from build123d import *

# Parameters (mm, degrees)
SKETCH1_R                   = 13
BOSS_EXTRUDE1_DEPTH         = 3.5
SKETCH2_R                   = 20
BOSS_EXTRUDE2_DEPTH         = 1
SKETCH3_R                   = 26
BOSS_EXTRUDE3_DEPTH         = 1
SKETCH4_R                   = 23.03
BOSS_EXTRUDE4_DEPTH         = 7.5
SKETCH5_R                   = 26
BOSS_EXTRUDE5_DEPTH         = 1
SKETCH6_R                   = 20
BOSS_EXTRUDE6_DEPTH         = 1
SKETCH7_R                   = 11
CUT_EXTRUDE1_DEPTH          = 40.711459303
TAP_DRILL_FOR_M3X0_5_TAP1_D = 3.4
CHAMFER1_SIZE               = 0.5


with BuildPart() as part:
    # Sketch1 → Boss-Extrude1 (new body)
    with BuildSketch(Plane.XY):
        Circle(SKETCH1_R)
    extrude(amount=BOSS_EXTRUDE1_DEPTH)

    # Sketch2 → Boss-Extrude2 (add)
    with BuildSketch(Plane.XY.offset(3.5)):
        Circle(SKETCH2_R)
    extrude(amount=BOSS_EXTRUDE2_DEPTH)

    # Sketch3 → Boss-Extrude3 (add)
    with BuildSketch(Plane.XY.offset(4.5)):
        Circle(SKETCH3_R)
    extrude(amount=BOSS_EXTRUDE3_DEPTH)

    # Sketch4 → Boss-Extrude4 (add)
    with BuildSketch(Plane.XY.offset(5.5)):
        Circle(SKETCH4_R)
    extrude(amount=BOSS_EXTRUDE4_DEPTH)

    # Sketch5 → Boss-Extrude5 (add)
    with BuildSketch(Plane.XY.offset(13)):
        Circle(SKETCH5_R)
    extrude(amount=BOSS_EXTRUDE5_DEPTH)

    # Sketch6 → Boss-Extrude6 (add)
    with BuildSketch(Plane.XY.offset(14)):
        Circle(SKETCH6_R)
    extrude(amount=BOSS_EXTRUDE6_DEPTH)

    # Sketch7 → Cut-Extrude1 (cut, through all)
    with BuildSketch(Plane.XY.offset(15)):
        Circle(SKETCH7_R)
    extrude(amount=-CUT_EXTRUDE1_DEPTH, mode=Mode.SUBTRACT)

    # Tap Drill for M3x0.5 Tap1 (through all)
    with Locations(Plane(origin=(0, 0, 3.5), x_dir=(-1, 0, 0), z_dir=(0, 0, -1))):
        with Locations((0, 17), (17, 0), (0, -17), (-17, 0)):
            Hole(TAP_DRILL_FOR_M3X0_5_TAP1_D / 2)

    # Chamfer1
    chamfer1_edges = [part.edges().sort_by_distance(p)[0] for p in [
        (-20, 0, 15),
    ]]
    chamfer(chamfer1_edges, length=CHAMFER1_SIZE)


solid = part.part
Source: CAD feature listing. Evaluate the final solid. Frame: model axes, mm. A direction names the side the tool comes from. Coordinates: 2 decimals unless noted, no trailing zeros. Order: outer loops, then holes, each group sorted by start corner. A loop starts at its lowest first (then second) coordinate and runs counter-clockwise, first axis right, second up.
Item 1: Cut plane B-B (y = 0). Count the separate pieces of the cut face and the enclosed holes in it, plus the area to 3 significant figures.
Output values:
separate pieces: 4
enclosed holes: 0
area: 212 mm2
Item 2: Set-up query: faces 5 (the face through (-10.316, -7.91, 1.726)), 6 (the face through (-4.336, -19.524, 14.246)), 7 (the face through (-16, -17, 13)). Return all of +Z, -Z, +X, -X, +Y, -Y with unobstructed straight access to the full face (end or side cutting, diameter ignored); none if empty.
Output values:
face 5: -Z
face 6: +Z
face 7: none
Item 3: Pull-direction query (Z, two-part tool) for faces 1 (the face through (-16, -17, 5.5)), 2 (the face through (4, -13, 3.5)), 3 (the face through (-0.221, 18.686, 9.33)), 4 (the face through (-4.992, -22.482, 9.198)); classes: pulls with the +Z half, pulls with the -Z half, needs draft (parallel to the pull), parting line crosses it, or undercut.
Output values:
face 1: undercut
face 2: pulls with the -Z half
face 3: needs draft
face 4: undercut
Item 4: Cut plane A-A (z = 7). Return loops of the section in (x, y).
Output values:
outline: circle Ø46.06 at (0, 0); hole circle Ø3.4 at (-17, 0); hole circle Ø22 at (0, 0); hole circle Ø3.4 at (0, -17); hole circle Ø3.4 at (0, 17); hole circle Ø3.4 at (17, 0)
Item 5: Material intervals for line 1 (Y direction, x = 0, z = 9.75); line 2 (Z direction, x = 11.5, y = 23); line 3 (Y direction, x = -10, z = 13.75), sorted ascending.
Output values:
line 1: y = -23.03 to -18.7, -15.3 to -11, 11 to 15.3, 18.7 to 23.03
line 2: z = 4.5 to 5.5, 13 to 14
line 3: y = -24 to -4.58, 4.58 to 24
Item 6: First-contact query: P1, Ø1, axis at x = 17, y = 15, coming from the +Z side; P2, Ø1.5, axis at x = -15.5, z = 6.5, coming from the +Y side; P3, Ø1.5, axis at y = 19, z = 9.5, coming from the +X side. Flat tips, straight axial feed; report the tip coordinate or a pass-through.
Output values:
P1: stops at z = 14
P2: stops at y = 17.69
P3: stops at x = 14.05
